from build123d import *

# Parameters (mm, degrees)
SKETCH1_W                   = 50.8
SKETCH1_H                   = 50.8
SKETCH1_W_2                 = 44.45
SKETCH1_H_2                 = 44.45
BOSS_EXTRUDE1_DEPTH         = 546.1
CUT_EXTRUDE1_REACH          = 552.805
SKETCH2_R                   = 2.4638
CUT_EXTRUDE2_REACH          = 552.805
SKETCH3_R                   = 2.4638
F_1_4_0_25_DIAMETER_HOLE1_D = 6.746875
CUT_EXTRUDE3_REACH          = 552.805
SKETCH10_R                  = 2.579751
SKETCH10_R_2                = 2.61565382
SKETCH12_R                  = 3.3734375
CUT_EXTRUDE4_DEPTH          = 551.805310432
CUT_EXTRUDE5_REACH          = 552.805
SKETCH13_R                  = 2.5796875
SKETCH14_R                  = 3.3734375
CUT_EXTRUDE6_DEPTH          = 551.805310432
CUT_EXTRUDE7_REACH          = 552.805
SKETCH15_R                  = 6.35


with BuildPart() as part:
    # Sketch1 → Boss-Extrude1 (new body)
    with BuildSketch(Plane(origin=(0, 0, 0), x_dir=(1, 0, 0), z_dir=(0, 1, 0))):
        with Locations((25.4, 25.4)):
            Rectangle(SKETCH1_W, SKETCH1_H)
        with Locations((25.4, 25.4)):
            Rectangle(SKETCH1_W_2, SKETCH1_H_2, mode=Mode.SUBTRACT)
    extrude(amount=BOSS_EXTRUDE1_DEPTH)

    # Sketch2 → Cut-Extrude1 (cut, up to next)
    with BuildSketch(Plane.XY, mode=Mode.PRIVATE) as cut_extrude1_sk1:
        with Locations((38.1, 12.7)):
            Circle(SKETCH2_R)
    cut_extrude1_tool1 = extrude(cut_extrude1_sk1.sketch, amount=-CUT_EXTRUDE1_REACH, mode=Mode.PRIVATE) & part.part
    # Sketch2 → Cut-Extrude1 (cut, up to next)
    with BuildSketch(Plane.XY, mode=Mode.PRIVATE) as cut_extrude1_sk2:
        with Locations((12.7, 12.7)):
            Circle(SKETCH2_R)
    cut_extrude1_tool2 = extrude(cut_extrude1_sk2.sketch, amount=-CUT_EXTRUDE1_REACH, mode=Mode.PRIVATE) & part.part
    # Sketch2 → Cut-Extrude1 (cut, up to next)
    with BuildSketch(Plane.XY, mode=Mode.PRIVATE) as cut_extrude1_sk3:
        with Locations((12.7, 50.8)):
            Circle(SKETCH2_R)
    cut_extrude1_tool3 = extrude(cut_extrude1_sk3.sketch, amount=-CUT_EXTRUDE1_REACH, mode=Mode.PRIVATE) & part.part
    # Sketch2 → Cut-Extrude1 (cut, up to next)
    with BuildSketch(Plane.XY, mode=Mode.PRIVATE) as cut_extrude1_sk4:
        with Locations((38.1, 50.8)):
            Circle(SKETCH2_R)
    cut_extrude1_tool4 = extrude(cut_extrude1_sk4.sketch, amount=-CUT_EXTRUDE1_REACH, mode=Mode.PRIVATE) & part.part
    # Sketch2 → Cut-Extrude1 (cut, up to next)
    with BuildSketch(Plane.XY, mode=Mode.PRIVATE) as cut_extrude1_sk5:
        with Locations((38.1, 495.3)):
            Circle(SKETCH2_R)
    cut_extrude1_tool5 = extrude(cut_extrude1_sk5.sketch, amount=-CUT_EXTRUDE1_REACH, mode=Mode.PRIVATE) & part.part
    # Sketch2 → Cut-Extrude1 (cut, up to next)
    with BuildSketch(Plane.XY, mode=Mode.PRIVATE) as cut_extrude1_sk6:
        with Locations((12.7, 495.3)):
            Circle(SKETCH2_R)
    cut_extrude1_tool6 = extrude(cut_extrude1_sk6.sketch, amount=-CUT_EXTRUDE1_REACH, mode=Mode.PRIVATE) & part.part
    # Sketch2 → Cut-Extrude1 (cut, up to next)
    with BuildSketch(Plane.XY, mode=Mode.PRIVATE) as cut_extrude1_sk7:
        with Locations((12.7, 533.4)):
            Circle(SKETCH2_R)
    cut_extrude1_tool7 = extrude(cut_extrude1_sk7.sketch, amount=-CUT_EXTRUDE1_REACH, mode=Mode.PRIVATE) & part.part
    # Sketch2 → Cut-Extrude1 (cut, up to next)
    with BuildSketch(Plane.XY, mode=Mode.PRIVATE) as cut_extrude1_sk8:
        with Locations((38.1, 533.4)):
            Circle(SKETCH2_R)
    cut_extrude1_tool8 = extrude(cut_extrude1_sk8.sketch, amount=-CUT_EXTRUDE1_REACH, mode=Mode.PRIVATE) & part.part
    add(cut_extrude1_tool1.solids().sort_by_distance((38.1, 12.7, 0))[0], mode=Mode.SUBTRACT)
    add(cut_extrude1_tool2.solids().sort_by_distance((12.7, 12.7, 0))[0], mode=Mode.SUBTRACT)
    add(cut_extrude1_tool3.solids().sort_by_distance((12.7, 50.8, 0))[0], mode=Mode.SUBTRACT)
    add(cut_extrude1_tool4.solids().sort_by_distance((38.1, 50.8, 0))[0], mode=Mode.SUBTRACT)
    add(cut_extrude1_tool5.solids().sort_by_distance((38.1, 495.3, 0))[0], mode=Mode.SUBTRACT)
    add(cut_extrude1_tool6.solids().sort_by_distance((12.7, 495.3, 0))[0], mode=Mode.SUBTRACT)
    add(cut_extrude1_tool7.solids().sort_by_distance((12.7, 533.4, 0))[0], mode=Mode.SUBTRACT)
    add(cut_extrude1_tool8.solids().sort_by_distance((38.1, 533.4, 0))[0], mode=Mode.SUBTRACT)

    # Sketch3 → Cut-Extrude2 (cut, up to next)
    with BuildSketch(Plane(origin=(0, 0, -50.8), x_dir=(-1, 0, 0), z_dir=(0, 0, -1)), mode=Mode.PRIVATE) as cut_extrude2_sk1:
        with Locations(Location((-38.1, 533.4, 0), (0, 0, 180))):
            Circle(SKETCH3_R)
    cut_extrude2_tool1 = extrude(cut_extrude2_sk1.sketch, amount=-CUT_EXTRUDE2_REACH, mode=Mode.PRIVATE) & part.part
    # Sketch3 → Cut-Extrude2 (cut, up to next)
    with BuildSketch(Plane(origin=(0, 0, -50.8), x_dir=(-1, 0, 0), z_dir=(0, 0, -1)), mode=Mode.PRIVATE) as cut_extrude2_sk2:
        with Locations(Location((-12.7, 533.4, 0), (0, 0, 180))):
            Circle(SKETCH3_R)
    cut_extrude2_tool2 = extrude(cut_extrude2_sk2.sketch, amount=-CUT_EXTRUDE2_REACH, mode=Mode.PRIVATE) & part.part
    # Sketch3 → Cut-Extrude2 (cut, up to next)
    with BuildSketch(Plane(origin=(0, 0, -50.8), x_dir=(-1, 0, 0), z_dir=(0, 0, -1)), mode=Mode.PRIVATE) as cut_extrude2_sk3:
        with Locations((-38.1, 429.26)):
            Circle(SKETCH3_R)
    cut_extrude2_tool3 = extrude(cut_extrude2_sk3.sketch, amount=-CUT_EXTRUDE2_REACH, mode=Mode.PRIVATE) & part.part
    # Sketch3 → Cut-Extrude2 (cut, up to next)
    with BuildSketch(Plane(origin=(0, 0, -50.8), x_dir=(-1, 0, 0), z_dir=(0, 0, -1)), mode=Mode.PRIVATE) as cut_extrude2_sk4:
        with Locations((-12.7, 429.26)):
            Circle(SKETCH3_R)
    cut_extrude2_tool4 = extrude(cut_extrude2_sk4.sketch, amount=-CUT_EXTRUDE2_REACH, mode=Mode.PRIVATE) & part.part
    # Sketch3 → Cut-Extrude2 (cut, up to next)
    with BuildSketch(Plane(origin=(0, 0, -50.8), x_dir=(-1, 0, 0), z_dir=(0, 0, -1)), mode=Mode.PRIVATE) as cut_extrude2_sk5:
        with Locations((-38.1, 325.12)):
            Circle(SKETCH3_R)
    cut_extrude2_tool5 = extrude(cut_extrude2_sk5.sketch, amount=-CUT_EXTRUDE2_REACH, mode=Mode.PRIVATE) & part.part
    # Sketch3 → Cut-Extrude2 (cut, up to next)
    with BuildSketch(Plane(origin=(0, 0, -50.8), x_dir=(-1, 0, 0), z_dir=(0, 0, -1)), mode=Mode.PRIVATE) as cut_extrude2_sk6:
        with Locations((-12.7, 325.12)):
            Circle(SKETCH3_R)
    cut_extrude2_tool6 = extrude(cut_extrude2_sk6.sketch, amount=-CUT_EXTRUDE2_REACH, mode=Mode.PRIVATE) & part.part
    # Sketch3 → Cut-Extrude2 (cut, up to next)
    with BuildSketch(Plane(origin=(0, 0, -50.8), x_dir=(-1, 0, 0), z_dir=(0, 0, -1)), mode=Mode.PRIVATE) as cut_extrude2_sk7:
        with Locations((-38.1, 220.98)):
            Circle(SKETCH3_R)
    cut_extrude2_tool7 = extrude(cut_extrude2_sk7.sketch, amount=-CUT_EXTRUDE2_REACH, mode=Mode.PRIVATE) & part.part
    # Sketch3 → Cut-Extrude2 (cut, up to next)
    with BuildSketch(Plane(origin=(0, 0, -50.8), x_dir=(-1, 0, 0), z_dir=(0, 0, -1)), mode=Mode.PRIVATE) as cut_extrude2_sk8:
        with Locations((-12.7, 220.98)):
            Circle(SKETCH3_R)
    cut_extrude2_tool8 = extrude(cut_extrude2_sk8.sketch, amount=-CUT_EXTRUDE2_REACH, mode=Mode.PRIVATE) & part.part
    # Sketch3 → Cut-Extrude2 (cut, up to next)
    with BuildSketch(Plane(origin=(0, 0, -50.8), x_dir=(-1, 0, 0), z_dir=(0, 0, -1)), mode=Mode.PRIVATE) as cut_extrude2_sk9:
        with Locations((-38.1, 116.84)):
            Circle(SKETCH3_R)
    cut_extrude2_tool9 = extrude(cut_extrude2_sk9.sketch, amount=-CUT_EXTRUDE2_REACH, mode=Mode.PRIVATE) & part.part
    # Sketch3 → Cut-Extrude2 (cut, up to next)
    with BuildSketch(Plane(origin=(0, 0, -50.8), x_dir=(-1, 0, 0), z_dir=(0, 0, -1)), mode=Mode.PRIVATE) as cut_extrude2_sk10:
        with Locations((-12.7, 116.84)):
            Circle(SKETCH3_R)
    cut_extrude2_tool10 = extrude(cut_extrude2_sk10.sketch, amount=-CUT_EXTRUDE2_REACH, mode=Mode.PRIVATE) & part.part
    # Sketch3 → Cut-Extrude2 (cut, up to next)
    with BuildSketch(Plane(origin=(0, 0, -50.8), x_dir=(-1, 0, 0), z_dir=(0, 0, -1)), mode=Mode.PRIVATE) as cut_extrude2_sk11:
        with Locations(Location((-38.1, 12.7, 0), (0, 0, 180))):
            Circle(SKETCH3_R)
    cut_extrude2_tool11 = extrude(cut_extrude2_sk11.sketch, amount=-CUT_EXTRUDE2_REACH, mode=Mode.PRIVATE) & part.part
    # Sketch3 → Cut-Extrude2 (cut, up to next)
    with BuildSketch(Plane(origin=(0, 0, -50.8), x_dir=(-1, 0, 0), z_dir=(0, 0, -1)), mode=Mode.PRIVATE) as cut_extrude2_sk12:
        with Locations(Location((-12.7, 12.7, 0), (0, 0, 180))):
            Circle(SKETCH3_R)
    cut_extrude2_tool12 = extrude(cut_extrude2_sk12.sketch, amount=-CUT_EXTRUDE2_REACH, mode=Mode.PRIVATE) & part.part
    add(cut_extrude2_tool1.solids().sort_by_distance((38.1, 533.4, -50.8))[0], mode=Mode.SUBTRACT)
    add(cut_extrude2_tool2.solids().sort_by_distance((12.7, 533.4, -50.8))[0], mode=Mode.SUBTRACT)
    add(cut_extrude2_tool3.solids().sort_by_distance((38.1, 429.26, -50.8))[0], mode=Mode.SUBTRACT)
    add(cut_extrude2_tool4.solids().sort_by_distance((12.7, 429.26, -50.8))[0], mode=Mode.SUBTRACT)
    add(cut_extrude2_tool5.solids().sort_by_distance((38.1, 325.12, -50.8))[0], mode=Mode.SUBTRACT)
    add(cut_extrude2_tool6.solids().sort_by_distance((12.7, 325.12, -50.8))[0], mode=Mode.SUBTRACT)
    add(cut_extrude2_tool7.solids().sort_by_distance((38.1, 220.98, -50.8))[0], mode=Mode.SUBTRACT)
    add(cut_extrude2_tool8.solids().sort_by_distance((12.7, 220.98, -50.8))[0], mode=Mode.SUBTRACT)
    add(cut_extrude2_tool9.solids().sort_by_distance((38.1, 116.84, -50.8))[0], mode=Mode.SUBTRACT)
    add(cut_extrude2_tool10.solids().sort_by_distance((12.7, 116.84, -50.8))[0], mode=Mode.SUBTRACT)
    add(cut_extrude2_tool11.solids().sort_by_distance((38.1, 12.7, -50.8))[0], mode=Mode.SUBTRACT)
    add(cut_extrude2_tool12.solids().sort_by_distance((12.7, 12.7, -50.8))[0], mode=Mode.SUBTRACT)

    # 1/4 (0.25) Diameter Hole1 (through all)
    with Locations(Plane(origin=(50.8, 0, 0), x_dir=(0, 0, -1), z_dir=(1, 0, 0))):
        with Locations((12.7, 482.6), (38.1, 482.6)):
            Hole(F_1_4_0_25_DIAMETER_HOLE1_D / 2)

    # Sketch10 → Cut-Extrude3 (cut, up to next)
    with BuildSketch(Plane.ZY, mode=Mode.PRIVATE) as cut_extrude3_sk1:
        with Locations((-7.62, 356.241430513)):
            Circle(SKETCH10_R)
    cut_extrude3_tool1 = extrude(cut_extrude3_sk1.sketch, amount=-CUT_EXTRUDE3_REACH, mode=Mode.PRIVATE) & part.part
    # Sketch10 → Cut-Extrude3 (cut, up to next)
    with BuildSketch(Plane.ZY, mode=Mode.PRIVATE) as cut_extrude3_sk2:
        with Locations((-7.62, 221.657333333)):
            Circle(SKETCH10_R_2)
    cut_extrude3_tool2 = extrude(cut_extrude3_sk2.sketch, amount=-CUT_EXTRUDE3_REACH, mode=Mode.PRIVATE) & part.part
    add(cut_extrude3_tool1.solids().sort_by_distance((0, 356.241431, -7.62))[0], mode=Mode.SUBTRACT)
    add(cut_extrude3_tool2.solids().sort_by_distance((0, 221.657333, -7.62))[0], mode=Mode.SUBTRACT)

    # Sketch12 → Cut-Extrude4 (cut, through all)
    with BuildSketch(Plane.ZY):
        with Locations((-12.7, 176.702529248)):
            Circle(SKETCH12_R)
        with Locations((-12.7, 125.902529248)):
            Circle(SKETCH12_R)
        with Locations((-38.1, 125.902529248)):
            Circle(SKETCH12_R)
        with Locations((-38.1, 176.702529248)):
            Circle(SKETCH12_R)
    extrude(amount=-CUT_EXTRUDE4_DEPTH, mode=Mode.SUBTRACT)

    # Sketch13 → Cut-Extrude5 (cut, up to next)
    with BuildSketch(Plane(origin=(50.8, 0, 0), x_dir=(0, 0, -1), z_dir=(1, 0, 0)), mode=Mode.PRIVATE) as cut_extrude5_sk1:
        with Locations((7.62, 379.321029287)):
            Circle(SKETCH13_R)
    cut_extrude5_tool1 = extrude(cut_extrude5_sk1.sketch, amount=-CUT_EXTRUDE5_REACH, mode=Mode.PRIVATE) & part.part
    # Sketch13 → Cut-Extrude5 (cut, up to next)
    with BuildSketch(Plane(origin=(50.8, 0, 0), x_dir=(0, 0, -1), z_dir=(1, 0, 0)), mode=Mode.PRIVATE) as cut_extrude5_sk2:
        with Locations((7.62, 74.521029287)):
            Circle(SKETCH13_R)
    cut_extrude5_tool2 = extrude(cut_extrude5_sk2.sketch, amount=-CUT_EXTRUDE5_REACH, mode=Mode.PRIVATE) & part.part
    add(cut_extrude5_tool1.solids().sort_by_distance((50.8, 379.321029, -7.62))[0], mode=Mode.SUBTRACT)
    add(cut_extrude5_tool2.solids().sort_by_distance((50.8, 74.521029, -7.62))[0], mode=Mode.SUBTRACT)

    # Sketch14 → Cut-Extrude6 (cut, through all)
    with BuildSketch(Plane.XY):
        with Locations((12.7, 80.518)):
            Circle(SKETCH14_R)
        with Locations((38.1, 80.518)):
            Circle(SKETCH14_R)
    extrude(amount=-CUT_EXTRUDE6_DEPTH, mode=Mode.SUBTRACT)

    # Sketch15 → Cut-Extrude7 (cut, up to next)
    with BuildSketch(Plane(origin=(0, 0, -50.8), x_dir=(-1, 0, 0), z_dir=(0, 0, -1)), mode=Mode.PRIVATE) as cut_extrude7_sk1:
        with Locations((-38.1, 80.518)):
            Circle(SKETCH15_R)
    cut_extrude7_tool1 = extrude(cut_extrude7_sk1.sketch, amount=-CUT_EXTRUDE7_REACH, mode=Mode.PRIVATE) & part.part
    # Sketch15 → Cut-Extrude7 (cut, up to next)
    with BuildSketch(Plane(origin=(0, 0, -50.8), x_dir=(-1, 0, 0), z_dir=(0, 0, -1)), mode=Mode.PRIVATE) as cut_extrude7_sk2:
        with Locations((-12.7, 80.518)):
            Circle(SKETCH15_R)
    cut_extrude7_tool2 = extrude(cut_extrude7_sk2.sketch, amount=-CUT_EXTRUDE7_REACH, mode=Mode.PRIVATE) & part.part
    add(cut_extrude7_tool1.solids().sort_by_distance((38.1, 80.518, -50.8))[0], mode=Mode.SUBTRACT)
    add(cut_extrude7_tool2.solids().sort_by_distance((12.7, 80.518, -50.8))[0], mode=Mode.SUBTRACT)


solid = part.part
The model under review builds one solid part; all positions refer to its coordinate system, in mm. A direction names the side the tool comes from. Round coordinates to 2 decimals unless told otherwise and drop trailing zeros. Loops run counter-clockwise (first coordinate to the right, second up) from the corner with the lowest first, then second, coordinate; pieces in that order, holes last. Notation, with made-up numbers: (35, 56) -> (73, 56) arc R5 cw to (73, 60) -> close; hole circle Ø10 at (62.5, 22.5). An arc over 180 degrees is marked (long way). One line per question, with ' | ' between items. Start each with the question number.
Item 1: Wall thickness on line 1 along X through (y, z) = (429, -50); line 2 along Y through (x, z) = (48.8, -38.1); line 3 along Y through (x, z) = (38.1, -2.4): over which ranges is each line inside the solid? List them lowest first. Write a range as [from, to].
Item 2: Draft analysis for pull direction Y (two halves, no side actions). For faces 1 (the face through (14.08, 74.32, -49.23)), 2 (the face through (25, 269, -47.625)), 3 (the face through (3, 546.1, -26)), state which applies: +Y half, -Y half, draft (parallel to the pull), parting line (faces both ways), or undercut.
Item 3: Add section B-B, the plane y = 258. Write out the cut boundary in (x, z) (3 decimals), then the cut area to 3 significant figures.
Item 4: For pin 1 (1.5 mm diameter, centred on x = 25.5, y = 225, fed in from +Z); pin 2 (12 mm diameter, centred on x = 30.5, z = -41.5, fed in from -Y), all flat-tipped, find the tip position at first contact; note any pin that passes through.
Item 5: Machinability: for faces 4 (the face through (3.175, 269, -25)), 5 (the face through (39.48, 74.32, -49.23)), 6 (the face through (25, 269, -50.8)), which of the approach directions +Z, -Z, +X, -X, +Y, -Y give a long, thin tool a straight path to every point of the face, cutting with its end or side? Answer none if there is none.
Item 6: Add section C-C, the plane z = -24. Write out the cut boundary in (x, y) (3 decimals), then the cut area to 3 significant figures.
Item 7: Add section A-A, the plane x = 25.5. Write out the cut boundary in (y, z) (3 decimals), then the cut area to 3 significant figures.
Return value:
1) line 1: x = [0, 10.25], [15.15, 35.65], [40.55, 50.8] | line 2: y = [0, 122.53], [129.28, 173.33], [180.08, 479.23], [485.97, 546.1] | line 3: y = [0, 10.24], [15.16, 48.34], [53.26, 77.14], [83.89, 492.84], [497.76, 530.94], [535.86, 546.1]
2) face 1: undercut | face 2: draft | face 3: +Y half
3) outline: (0, -50.8) -> (50.8, -50.8) -> (50.8, 0) -> (0, 0) -> close; hole (3.175, -47.625) -> (47.625, -47.625) -> (47.625, -3.175) -> (3.175, -3.175) -> close | area: 605 mm2
4) pin 1: stops at z = 0 | pin 2: passes through
5) face 4: +Y, -Y | face 5: -Z | face 6: -Z, +X, -X, +Y, -Y
6) outline: (0, 0) -> (3.175, 0) -> (3.175, 546.1) -> (0, 546.1) -> close; (47.625, 0) -> (50.8, 0) -> (50.8, 546.1) -> (47.625, 546.1) -> close | area: 3,470 mm2
7) outline: (0, -50.8) -> (546.1, -50.8) -> (546.1, -47.625) -> (0, -47.625) -> close; (0, -3.175) -> (546.1, -3.175) -> (546.1, 0) -> (0, 0) -> close | area: 3,470 mm2
